The listing builds one solid part. Answer for the finished solid, in the listing's coordinates (mm). Face numbers are marked on the shaded views. A direction names the side the tool comes from. Give positions to 0.01 mm unless a question says otherwise; leave off trailing zeros. Loops run counter-clockwise (first coordinate to the right, second up) from the corner with the lowest first, then second, coordinate; pieces in that order, holes last. Notation, with made-up numbers: M 74,61.5 L 106,61.5 A31 ccw 106,87.5 Z; hole C 82.25,1 d1. An arc over 180 degrees is marked long. Use one line per item in the form item = value. Start each with the question number.
1. Straight lines are drawn through the part: line 1 (Z direction, x = -20, y = 7.5); line 2 (X direction, y = 1.75, z = 1); line 3 (X direction, y = 3.75, z = -3). For each, find the intervals that lie inside material, in ascending order. Write a range as from..to.
2. The part is cut by section C-C (y = 5.5). Write down the section's boundary in (x, z), and give its area (3 significant figures).
3. Each of these flat-tipped pins is pushed along its axis until it touches: pin 1 Ø4 at (x, z) = (-28, 15.5) entering from -Y; pin 2 Ø10.5 at (x, z) = (20, 0) entering from +Y. Where does it stop, or does it pass through?
4. The mould has two halves that part along Z. Classify the marked faces 3, 4 and 5: released by +Z, released by -Z, zero draft, split by the parting line, or undercut.
5. For the marked faces 1 and 2, determine the directions among +Z, -Z, +X, -X, +Y, -Y from which every point of the face is accessible in a straight line to the end or side of a thin tool.
6. The part is cut by section A-A (z = 0). Write down the section's boundary in (x, y).
7. The part is cut by section D-D (z = 6). Write down the section's boundary in (x, y), and give its area (3 significant figures).
8. The part is cut by section B-B (x = 0). Write down the section's boundary in (y, z), and give its area (3 significant figures).
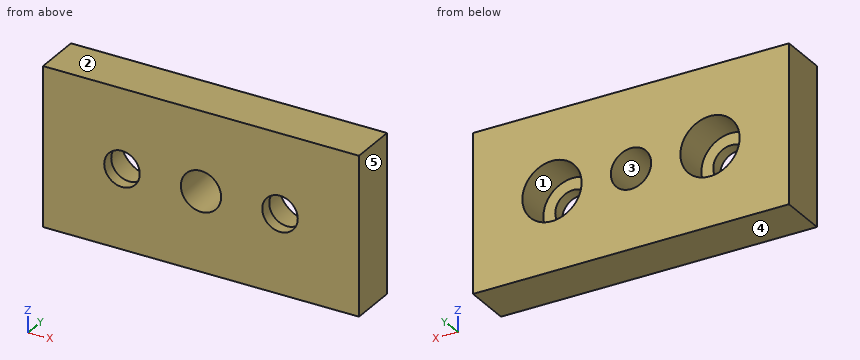
from build123d import *

# Parameters (mm, degrees)
SKETCH_1_W             = 80
SKETCH_1_H             = 40
EXTRUDE_1_DEPTH        = 12
HOLE_WIZARD_M121_D     = 10.2
HOLE_WIZARD_M121_DEPTH = 12


with BuildPart() as part:
    # Эскиз1 → Бобышка-Вытянуть1 (new body)
    with BuildSketch(Plane(origin=(0, 0, 0), x_dir=(1, 0, 0), z_dir=(0, 1, 0))):
        Rectangle(SKETCH_1_W, SKETCH_1_H)
    extrude(amount=EXTRUDE_1_DEPTH)

    # Эскиз2 → Вырез-Повернуть1 (revolve, cut)
    with BuildSketch(Plane.XY):
        Polygon((-27.5, 12), (-27.5, 3), (-24.5, 3), (-24.5, 0), (-20, 0), (-20, 12), align=None)
    cut_revolve_1 = revolve(axis=Axis((-20, 12, 0), (0, -1, 0)), mode=Mode.SUBTRACT)

    # Зеркальное отражение1: Вырез-Повернуть1 across plane
    add(cut_revolve_1.mirror(Plane(origin=(0, 0, 0), x_dir=(0, 0, 1), z_dir=(1, 0, 0))), mode=Mode.SUBTRACT)

    # Отверстие обработанное метчиком M121
    with Locations(Plane(origin=(0, 12, 0), x_dir=(1, 0, 0), z_dir=(0, 1, 0))):
        with Locations((0, 0)):
            Hole(HOLE_WIZARD_M121_D / 2, depth=HOLE_WIZARD_M121_DEPTH)


solid = part.part
Derived:
q1.line_1 = -20..-7.5, 7.5..20
q1.line_2 = -40..-24.39, -15.61..-5, 5..15.61, 24.39..40
q1.line_3 = -40..-26.87, -13.13..-4.12, 4.12..13.13, 26.87..40
q2.outline = M -40,-20 L 40,-20 L 40,20 L -40,20 Z; hole C -20,0 d15; hole C 0,0 d10.2; hole C 20,0 d15
q2.area = 2,760 mm2
q3.pin_1 = 0
q3.pin_2 = 3
q4.face_3 = undercut
q4.face_4 = released by -Z
q4.face_5 = zero draft
q5.face_1 = +Y
q5.face_2 = +Z, +X, -X, +Y, -Y
q6.outline = M -40,0 L -24.5,0 L -24.5,3 L -27.5,3 L -27.5,12 L -40,12 Z; M -15.5,0 L -5.1,0 L -5.1,12 L -12.5,12 L -12.5,3 L -15.5,3 Z; M 5.1,0 L 15.5,0 L 15.5,3 L 12.5,3 L 12.5,12 L 5.1,12 Z; M 24.5,0 L 40,0 L 40,12 L 27.5,12 L 27.5,3 L 24.5,3 Z
q7.outline = M -40,0 L 40,0 L 40,12 L 24.5,12 L 24.5,3 L 15.5,3 L 15.5,12 L -15.5,12 L -15.5,3 L -24.5,3 L -24.5,12 L -40,12 Z
q7.area = 798 mm2
q8.outline = M 0,-20 L 12,-20 L 12,-5.1 L 0,-5.1 Z; M 0,5.1 L 12,5.1 L 12,20 L 0,20 Z
q8.area = 358 mm2
